The model under review builds one solid part; all positions refer to its coordinate system, in mm. Face numbers are marked on the shaded views. A direction names the side the tool comes from. Coordinates: 2 decimals unless noted, no trailing zeros. Write each loop counter-clockwise with the first axis right and the second up, starting at its lowest first coordinate (ties: lowest second). Pieces come first, ordered by that corner, then holes.
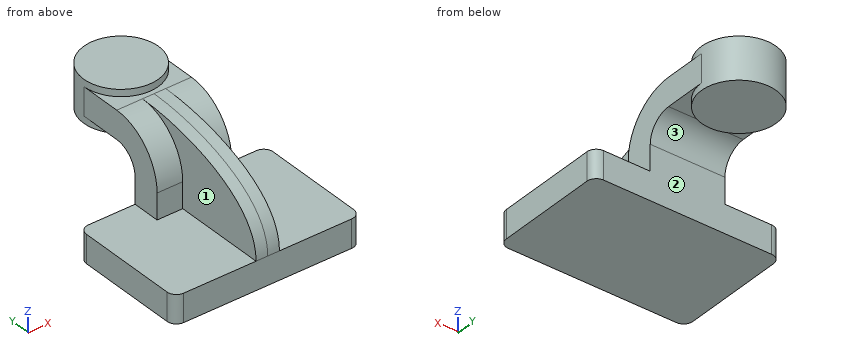
```python
from build123d import *

# Parameters (mm, degrees)
F1_DEPTH = 63.5
F0_W     = 25.4
F0_H     = 19.05
F2_DEPTH = 25.4
F3_DEPTH = 7.9375
F5_R     = 6.35


with BuildPart() as f1:
    # F0 (on Right) → F1 (new body, symmetric)
    with BuildSketch(Plane.YZ):
        Polygon((-41.275, -9.525), (41.275, -9.525), (41.275, 9.525), (22.225, 9.525), (-41.275, 9.525), align=None)
    extrude(amount=F1_DEPTH, both=True)

    # F0 (on Right) → F2 (join, symmetric)
    with BuildSketch(Plane.YZ):
        with BuildLine():
            Line((22.225, 9.525), (41.275, 9.525))
            Line((41.275, 9.525), (41.275, 27.0002))
            ThreePointArc((41.275, 27.0002), (45.9246798487, 38.2255201513), (57.15, 42.8752))
            Line((57.15, 42.8752), (60.325, 42.8752))
            Line((60.325, 42.8752), (60.325, 61.9252))
            Line((60.325, 61.9252), (57.15, 61.9252))
            ThreePointArc((57.15, 61.9252), (32.4542956671, 51.6959043329), (22.225, 27.0002))
            Line((22.225, 27.0002), (22.225, 9.525))
        make_face()
        with Locations((73.025, 52.4002)):
            Rectangle(F0_W, F0_H)
    extrude(amount=F2_DEPTH, both=True)

    # F0 (on Right) → F3 (join, symmetric)
    with BuildSketch(Plane.YZ):
        with BuildLine():
            add(Edge.make_bspline(
                [(57.15, 61.9252), (20.7915678899, 61.9252), (-41.275, 48.0412916491), (-41.275, 9.525)],
                knots=[0, 0, 0, 0, 111.5045361635, 111.5045361635, 111.5045361635, 111.5045361635], degree=3))
            Line((-41.275, 9.525), (22.225, 9.525))
            Line((22.225, 9.525), (22.225, 27.0002))
            ThreePointArc((22.225, 27.0002), (32.4542956671, 51.6959043329), (57.15, 61.9252))
        make_face()
    extrude(amount=F3_DEPTH, both=True)

    # F0 (on Right) → F4 (revolve)
    with BuildSketch(Plane.YZ):
        Polygon((85.725, 66.675), (85.725, 61.9252), (85.725, 42.8752), (85.725, 38.1), (111.125, 38.1), (111.125, 66.675), align=None)
    revolve(axis=Axis((0, 85.725, 52.3875), (0, 0, -1)))

    # F5
    f5_edges = [f1.edges().sort_by_distance(p)[0] for p in [
        (63.5, 41.275, 0),
        (63.5, -41.275, 0),
        (-63.5, -41.275, 0),
        (-63.5, 41.275, 0),
    ]]
    fillet(f5_edges, radius=F5_R)


solid = f1.part
```
Item 1: Take a section at D-D, the plane y = 83. Write out the cut boundary in (x, z) (3 decimals), plus the area to 3 significant figures.
Solved:
outline: (-25.4, 42.875) - (-25.253, 42.875) - (-25.253, 38.1) - (25.253, 38.1) - (25.253, 42.875) - (25.4, 42.875) - (25.4, 61.925) - (25.253, 61.925) - (25.253, 66.675) - (-25.253, 66.675) - (-25.253, 61.925) - (-25.4, 61.925) - close
area: 1,450 mm2
Item 2: Take a section at B-B, the plane y = 65. Write out the cut boundary in (x, z) (1 decimal).
Solved:
outline: (-25.4, 42.9) - (-14.7, 42.9) - (-14.7, 38.1) - (14.7, 38.1) - (14.7, 42.9) - (25.4, 42.9) - (25.4, 61.9) - (14.7, 61.9) - (14.7, 66.7) - (-14.7, 66.7) - (-14.7, 61.9) - (-25.4, 61.9) - close
Item 3: Take a section at A-A, the plane z = 6.5. Write out the cut boundary in (x, y) (3 decimals).
Solved:
outline: (-63.5, -34.925) arc R6.35 ccw to (-57.15, -41.275) - (57.15, -41.275) arc R6.35 ccw to (63.5, -34.925) - (63.5, 34.925) arc R6.35 ccw to (57.15, 41.275) - (-57.15, 41.275) arc R6.35 ccw to (-63.5, 34.925) - close
Item 4: Take a section at C-C, the plane x = 19. Write out the cut boundary in (y, z) (3 decimals).
Solved:
outline: (-41.275, -9.525) - (41.275, -9.525) - (41.275, 27) arc R15.875 cw to (57.15, 42.875) - (68.868, 42.875) - (68.868, 38.1) - (102.582, 38.1) - (102.582, 66.675) - (68.868, 66.675) - (68.868, 61.925) - (57.15, 61.925) arc R34.925 ccw to (22.225, 27) - (22.225, 9.525) - (-41.275, 9.525) - close
Item 5: Machinability: for the marked faces 1, 2 and 3, which of the approach directions +Z, -Z, +X, -X, +Y, -Y give a long, thin tool a straight path to every point of the face, cutting with its end or side? Answer none if there is none.
Solved:
face 1: +Z, -X, -Y
face 2: -Z, +X, -X, +Y
face 3: -Z, +X, -X
Item 6: For pin 1 (15.5 mm diameter, centred on y = 6.5, z = 27, fed in from +X); pin 2 (14.5 mm diameter, centred on x = -1, y = 77.5, fed in from -Z); pin 3 (2 mm diameter, centred on x = 25.5, z = 34, fed in from -Y), all flat-tipped, find the tip position at first contact; note any pin that passes through.
Solved:
pin 1: stops at x = 7.94
pin 2: stops at z = 38.1
pin 3: stops at y = 22.75
Item 7: To check wall thickness, follow line 1 along Z through (x, y) = (50, 33) (3 decimals); line 2 along X through (y, z) = (42, 36); line 3 along Y through (x, z) = (7, 38.5). State the ranges of each line that lie inside material, in increasing order.
Solved:
line 1: z = -9.525 to 9.525
line 2: x = -25.4 to 25.4
line 3: y = -26.07 to 46.21, 61.31 to 110.14
